Work out the finished part from the listing and answer in its coordinate system (mm). Give positions to 0.01 mm unless a question says otherwise; leave off trailing zeros. Loops run counter-clockwise (first coordinate to the right, second up) from the corner with the lowest first, then second, coordinate; pieces in that order, holes last. Notation, with made-up numbers: (9, 35) - (57, 35) arc R21 ccw to (57, 54) - close; hole circle Ø6 at (-12, 40). An arc over 180 degrees is marked (long way). Use one line per item in the form item = value. Start each with the question number.
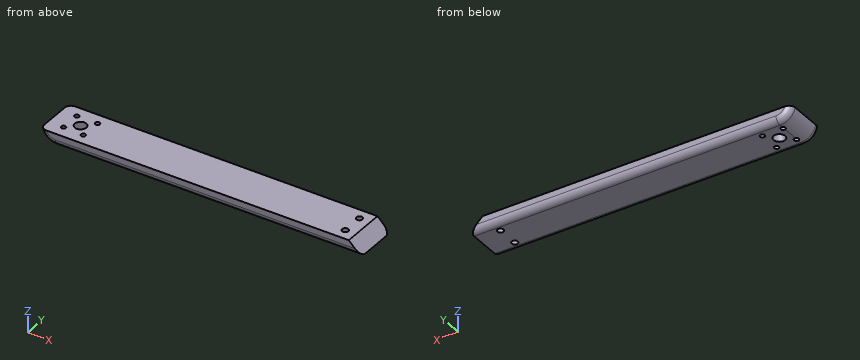
from build123d import *

# Parameters (mm, degrees)
ESQUISSE1_W             = 220
ESQUISSE1_H             = 28.284
BOSS_EXTRU_3_DEPTH      = 8
CHANFREIN1_SIZE         = 20
ESQUISSE4_R             = 2
ENL_V_MAT_EXTRU_1_DEPTH = 8
FILLET1_R               = 10
SKETCH2_R               = 1.5
SKETCH2_R_2             = 3.75
CUT_EXTRUDE1_DEPTH      = 8
FILLET4_R               = 4
FILLET5_R               = 4


with BuildPart() as part:
    # Esquisse1 → Boss.-Extru.3 (new body)
    with BuildSketch(Plane.XY):
        with Locations((110, 14.142)):
            Rectangle(ESQUISSE1_W, ESQUISSE1_H)
    extrude(amount=BOSS_EXTRU_3_DEPTH)

    # Chanfrein1
    # the kernel refuses this chamfer: 20 mm, written as the material it takes off along each edge
    with BuildSketch(Plane(origin=(220, -51.433659759, 8), x_dir=(0.027495876610586317, 0, -0.9996219169112968), z_dir=(0, 1, 0))) as chanfrein1_piece_1:
        Polygon((CHANFREIN1_SIZE * 0.999621916911, CHANFREIN1_SIZE * 0.0274958766106), (-CHANFREIN1_SIZE * 0.0274958766106, CHANFREIN1_SIZE * 0.999621916911), (0, 0), align=None)
    extrude(amount=131.151319519, mode=Mode.SUBTRACT)

    # Esquisse4 → Enlèv. mat.-Extru.1 (cut)
    with BuildSketch(Plane.XY.offset(8)):
        with Locations((193, 7.142)):
            Circle(ESQUISSE4_R)
        with Locations((193, 21.142)):
            Circle(ESQUISSE4_R)
    extrude(amount=-ENL_V_MAT_EXTRU_1_DEPTH, mode=Mode.SUBTRACT)

    # Fillet1
    # the kernel refuses this fillet: 10 mm, written as the material it takes off along each edge
    with BuildSketch(Plane(origin=(0, 52.778897428, 0), x_dir=(1, 0, 0), z_dir=(0, -1, 0))) as fillet1_piece_1:
        with BuildLine():
            CenterArc((9.797958971, 10), FILLET1_R, 191.536959033, 78.463040967)
            Line((0, 8), (-0.195959179, 7.96))
            ThreePointArc((-0.195959179, 7.96), (-0.2, 4), (-0.2, 0))
            Line((-0.2, 0), (0, -0.2))
            Line((0, -0.2), (9.797958971, -0.2))
            Line((9.797958971, -0.2), (9.797958971, 0))
        make_face()
    extrude(amount=77.273794856, mode=Mode.SUBTRACT)

    # Sketch2 → Cut-Extrude1 (cut)
    with BuildSketch(Plane.XY.offset(8)):
        with Locations((10.039316358, 7.799790773)):
            Circle(SKETCH2_R)
        with Locations((10.095797266, 20.845111475)):
            Circle(SKETCH2_R)
        with Locations((23.204777475, 7.243195633)):
            Circle(SKETCH2_R)
        with Locations((23.460536656, 20.883346587)):
            Circle(SKETCH2_R)
        with Locations((16.903459812, 14.177912334)):
            Circle(SKETCH2_R_2)
    extrude(amount=-CUT_EXTRUDE1_DEPTH, mode=Mode.SUBTRACT)

    # Fillet4
    fillet4_edges = [part.edges().sort_by_distance(p)[0] for p in [
        (108.898979486, 0, 0),
        (3.473403651, 0, 2.254033308),
    ]]
    fillet(fillet4_edges, radius=FILLET4_R)

    # Fillet5
    fillet5_edges = [part.edges().sort_by_distance(p)[0] for p in [
        (108.898979486, 28.284, 0),
        (3.473403651, 28.284, 2.254033308),
    ]]
    fillet(fillet5_edges, radius=FILLET5_R)


solid = part.part
1) Find the intervals of material crossed by probe 1 along Y at (x, z) = (193, 5.75); probe 2 along Y at (x, z) = (11, 4.25); probe 3 along X at (y, z) = (22, 7.25), in increasing order.
2) A cutting plane is placed at A-A (x = 193). Give the vertices of the cut face in (y, z), plus the area to 3 significant figures.
3) A flat-ended cylindrical pin translates along its axis: pin 1 Ø1.5 at (y, z) = (17.5, 7) entering from -X. Find the tip coordinate at first contact, or state that the pin passes through.
4) A cutting plane is placed at B-B (x = 122). Give the vertices of the cut face in (y, z).
5) A cutting plane is placed at C-C (z = 2.5). State how many separate pieces and enclosed holes the cut face has, plus the area to 3 significant figures.
Answer sheet:
q1.probe_1 = 0 to 5.14, 9.14 to 19.14, 23.14 to 28.28
q1.probe_2 = 0 to 6.65, 8.95 to 19.65, 22.04 to 28.28
q1.probe_3 = 0.18 to 9.14, 11.05 to 22.46, 24.46 to 191.19, 194.81 to 200.75
q2.outline = (0, 4) arc R4 ccw to (4, 0) - (5.14, 0) - (5.14, 8) - (0, 8) - close; (9.14, 0) - (19.14, 0) - (19.14, 8) - (9.14, 8) - close; (23.14, 0) - (24.28, 0) arc R4 ccw to (28.28, 4) - (28.28, 8) - (23.14, 8) - close
q2.area = 155 mm²
q3.pin_1 = 0.05
q4.outline = (0, 4) arc R4 ccw to (4, 0) - (24.28, 0) arc R4 ccw to (28.28, 4) - (28.28, 8) - (0, 8) - close
q5.separate_pieces = 1
q5.enclosed_holes = 7
q5.area = 5,500 mm²
